from build123d import *

# Parameters (mm, degrees)
CROQUIS2_W                 = 50
CROQUIS2_H                 = 25
SALIENTE_EXTRUIR2_DEPTH    = 25
CROQUIS9_W                 = 25
CROQUIS9_H                 = 25
SALIENTE_EXTRUIR3_DEPTH    = 50
CROQUIS10_R                = 8
CORTAR_EXTRUIR2_DEPTH      = 43
CORTAR_EXTRUIR2_DEPTH_BACK = 49
CROQUIS11_R                = 8
CORTAR_EXTRUIR3_DEPTH      = 37.5
REDONDEO1_R                = 5
SALIENTE_EXTRUIR4_DEPTH    = 12.5
CROQUIS15_R                = 2
CORTAR_EXTRUIR4_DEPTH      = 33
CROQUIS16_R                = 2
CORTAR_EXTRUIR5_DEPTH      = 33


with BuildPart() as part:
    # Croquis2 → Saliente-Extruir2 (new body)
    with BuildSketch(Plane(origin=(0, 0, 0), x_dir=(1, 0, 0), z_dir=(0, 1, 0))):
        Rectangle(CROQUIS2_W, CROQUIS2_H)
    extrude(amount=SALIENTE_EXTRUIR2_DEPTH)

    # Croquis9 → Saliente-Extruir3 (add)
    with BuildSketch(Plane(origin=(0, 0, 0), x_dir=(1, 0, 0), z_dir=(0, 1, 0))):
        Rectangle(CROQUIS9_W, CROQUIS9_H)
    extrude(amount=SALIENTE_EXTRUIR3_DEPTH)

    # Croquis10 → Cortar-Extruir2 (cut, two sides)
    with BuildSketch(Plane(origin=(0, 0, 0), x_dir=(0, 0, -1), z_dir=(1, 0, 0))) as cortar_extruir2_sk:
        with Locations((0, 12.957262023)):
            Circle(CROQUIS10_R)
    extrude(amount=CORTAR_EXTRUIR2_DEPTH, mode=Mode.SUBTRACT)
    extrude(cortar_extruir2_sk.sketch, amount=-CORTAR_EXTRUIR2_DEPTH_BACK, mode=Mode.SUBTRACT)

    # Croquis11 → Cortar-Extruir3 (cut, symmetric)
    with BuildSketch(Plane(origin=(0, 50, 0), x_dir=(1, 0, 0), z_dir=(0, 1, 0))):
        Circle(CROQUIS11_R)
    extrude(amount=CORTAR_EXTRUIR3_DEPTH, both=True, mode=Mode.SUBTRACT)

    # Redondeo1
    redondeo1_edges = [part.edges().sort_by_distance(p)[0] for p in [
        (12.5, 25, 0),
        (-12.5, 25, 0),
    ]]
    fillet(redondeo1_edges, radius=REDONDEO1_R)

    # Croquis13 → Saliente-Extruir4 (add, symmetric)
    with BuildSketch(Plane.XY):
        with BuildLine():
            Line((-25, 0), (25, 0))
            ThreePointArc((25, 0), (0, -4.006579232), (-25, 0))
        make_face()
    extrude(amount=SALIENTE_EXTRUIR4_DEPTH, both=True)

    # Croquis15 → Cortar-Extruir4 (cut)
    with BuildSketch(Plane.ZY.offset(12.5)):
        with Locations((0.568263939, 40.759281312)):
            Circle(CROQUIS15_R)
    extrude(amount=-CORTAR_EXTRUIR4_DEPTH, mode=Mode.SUBTRACT)

    # Croquis16 → Cortar-Extruir5 (cut)
    with BuildSketch(Plane(origin=(0, 25, 0), x_dir=(1, 0, 0), z_dir=(0, 1, 0))):
        with Locations((20.833740283, 0)):
            Circle(CROQUIS16_R)
    cortar_extruir5 = extrude(amount=-CORTAR_EXTRUIR5_DEPTH, mode=Mode.SUBTRACT)

    # Simetría1: Cortar-Extruir5 across plane
    add(cortar_extruir5.mirror(Plane(origin=(0, 0, 0), x_dir=(0, 0, 1), z_dir=(1, 0, 0))), mode=Mode.SUBTRACT)


solid = part.part
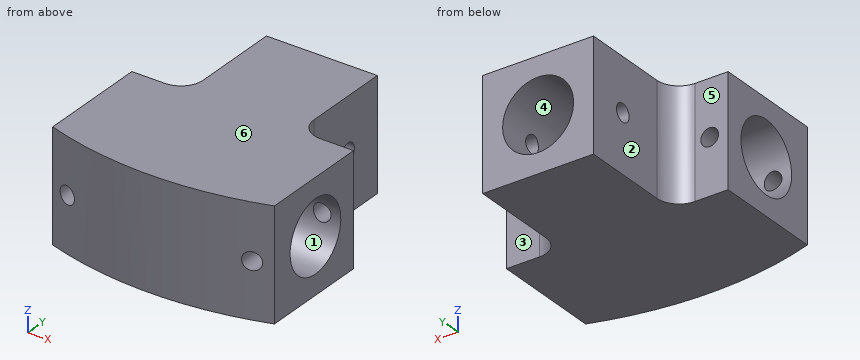
For this review, take the finished solid that the model builds, in its own axes (mm). Face numbers are marked on the shaded views. A direction names the side the tool comes from. Round coordinates to 2 decimals unless told otherwise and drop trailing zeros. Write each loop counter-clockwise with the first axis right and the second up, starting at its lowest first coordinate (ties: lowest second). Pieces come first, ordered by that corner, then holes. Notation, with made-up numbers: (71.5, 60) - (105.5, 60) arc R24 ccw to (105.5, 95) - close; hole circle Ø8 at (76.5, 70). An arc over 180 degrees is marked (long way). Use a Markdown table: item, result.
Q1. Machinability: for the marked faces 1, 2 and 3, which of the approach directions +Z, -Z, +X, -X, +Y, -Y give a long, thin tool a straight path to every point of the face, cutting with its end or side? Answer none if there is none.
Derived:
| item | result |
|---|---|
| face 1 | +X, -X |
| face 2 | +Z, -Z, -X, +Y |
| face 3 | +Z, -Z, +X, +Y |
Q2. We need section C-C (y = 17). Give the boundary of the cut face in (x, z).
Derived:
| item | result |
|---|---|
| outline | (-25, -12.5) - (25, -12.5) - (25, -6.9) - (4.04, -6.9) arc R8 cw to (-4.04, -6.9) - (-25, -6.9) - close; (-25, 6.9) - (-4.04, 6.9) arc R8 cw to (4.04, 6.9) - (25, 6.9) - (25, 12.5) - (-25, 12.5) - close |
Q3. The part is to be moulded in two halves that separate along Z. For the marked faces 4, 5 and 6, say which applies: pulls with the +Z half, pulls with the -Z half, needs draft (parallel to the pull), parting line crosses it, or undercut.
Derived:
| item | result |
|---|---|
| face 4 | undercut |
| face 5 | needs draft |
| face 6 | pulls with the +Z half |
Q4. We need section B-B (x = 16). Give the boundary of the cut face in (y, z).
Derived:
| item | result |
|---|---|
| outline | (-2.39, -12.5) - (25.23, -12.5) - (25.23, 12.5) - (-2.39, 12.5) - close; hole circle Ø16 at (12.96, 0) |
Q5. Wall thickness on line 1 along X through (y, z) = (24, 0); line 2 along X through (y, z) = (3.25, 0); line 3 along Y through (x, z) = (-11.5, 0): over which ranges is each line inside the solid? List them lowest first.
Derived:
| item | result |
|---|---|
| line 1 | x = -25 to -22.83, -18.83 to -8, 8 to 18.83, 22.83 to 25 |
| line 2 | x = -25 to -22.83, -18.83 to 18.83, 22.83 to 25 |
| line 3 | y = -3.18 to 4.96, 20.96 to 38.84, 42.68 to 50 |
Q6. We need section A-A (y = 33.5). Give the boundary of the cut face in (x, z).
Derived:
| item | result |
|---|---|
| outline | (-12.5, -12.5) - (12.5, -12.5) - (12.5, 12.5) - (-12.5, 12.5) - close; hole circle Ø16 at (0, 0) |
Q7. We need section D-D (z = 0). State how many separate pieces and enclosed holes the cut face has, plus the area to 3 significant figures.
Derived:
| item | result |
|---|---|
| separate pieces | 9 |
| enclosed holes | 0 |
| area | 639 mm2 |
Q8. Clearance check with flat-ended pins moving along their axes: pin 1 (8 mm diameter, centred on x = 1, z = -4, fed in from +Y); pin 2 (4.5 mm diameter, centred on x = 20.83, z = 0, fed in from +Y); pin 3 (5 mm diameter, centred on y = 40.76, z = 0.57, fed in from -X); pin 4 (14.5 mm diameter, centred on x = 0, z = 0, fed in from -Y). State where each tip first meets the part, or that it passes through.
Derived:
| item | result |
|---|---|
| pin 1 | stops at y = 50 |
| pin 2 | stops at y = 25 |
| pin 3 | stops at x = -12.5 |
| pin 4 | stops at y = -4.01 |
